Autodesk Inventor part; units mm, degrees
ref_plane "YZ Plane" through (0, 0, 0) normal (1, 0, 0) x (0, 1, 0)
ref_plane "XZ Plane" through (0, 0, 0) normal (0, 1, 0) x (-1, 0, 0)
ref_plane "XY Plane" through (0, 0, 0) normal (0, 0, 1) x (1, 0, 0)
sketch "スケッチ1" plane through (0, 0, 0) normal (0, 0, 1) x (1, 0, 0)
  circle A0 centre (0, 0) radius 1.5
  dimension "d0" = 3
extrude "押し出し1" add sketch "スケッチ1" along normal blind 4
sketch "スケッチ2" plane through (0, 0, 0) normal (0, 0, -1) x (-1, 0, 0)
  circle A0 centre (0, 0) radius 3
  dimension "d3" = 6
extrude "押し出し2" add sketch "スケッチ2" against normal blind 2
thread "ねじ1"
chamfer "面取り1" distance 1.5 angle 45 1 edges at (3, 0, 2)
properties part number "ネジ皿m3,04" material "鋼、高強度、低合金"
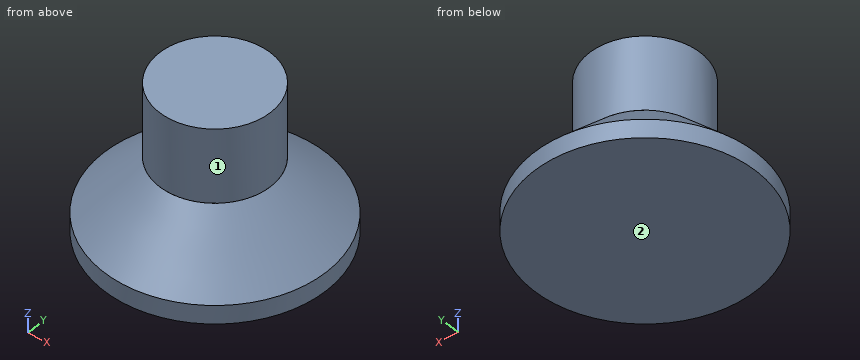
Verification items for the finished model (mm, model axes). Face numbers are marked on the shaded views. A direction names the side the tool comes from. Round coordinates to 2 decimals unless told otherwise and drop trailing zeros. Order: outer loops, then holes, each group sorted by start corner. A loop starts at its lowest first (then second) coordinate and runs counter-clockwise, first axis right, second up.
1) Material ranges on line 1 (Y direction, x = -0.8, z = 2.6); line 2 (X direction, y = 0.7, z = 0.8); line 3 (Y direction, x = 1.25, z = 1), recorded low to high.
Geometry says:
line 1: y = -1.27 to 1.27
line 2: x = -2.61 to 2.61
line 3: y = -2.17 to 2.17
2) Cross-section at D-D, the plane z = 1.85. Record the cut outline in (x, y), plus the area to 3 significant figures.
Geometry says:
outline: circle Ø3.3 at (0, 0)
area: 8.55 mm2
3) Cross-section at C-C, the plane z = 0.7. Record the cut outline in (x, y), plus the area to 3 significant figures.
Geometry says:
outline: circle Ø5.6 at (0, 0)
area: 24.6 mm2
4) Tool access check on the marked faces 1 and 2. Record the directions out of +Z, -Z, +X, -X, +Y, -Y that give a thin tool (end or side, any length) a straight path to the whole face; none if there is none.
Geometry says:
face 1: +Z
face 2: -Z, +X, -X, +Y, -Y
5) Depth check by flat-ended pin: pin 1 (1 mm diameter, centred on x = 0, z = 3, fed in from -Y). Enter the tip coordinate at first touch or a pass-through.
Geometry says:
pin 1: stops at y = -1.5
